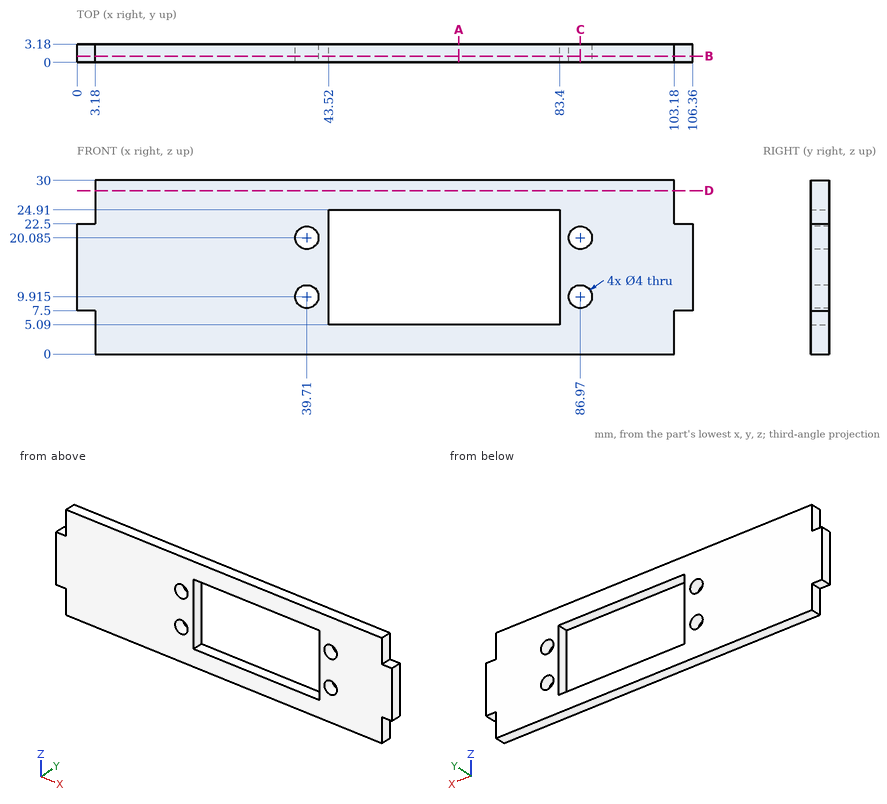
Part print with two shaded views. Sizes in mm from the minimum x, y, z corner. Round coordinates to 2 decimals unless told otherwise and drop trailing zeros. Order: outer loops, then holes, each group sorted by start corner. A loop starts at its lowest first (then second) coordinate and runs counter-clockwise, first axis right, second up.
(1) Band-saw the part on A-A (x = 66). List the corners of the cut face in (y, z).
(2) Band-saw the part on C-C (x = 86.97). List the corners of the cut face in (y, z) (3 decimals), then the cut area to 3 significant figures.
(3) Band-saw the part on D-D (z = 28.25). List the corners of the cut face in (x, y), then the cut area to 3 significant figures.
(4) Drill centre lines: line 1 (Z direction, x = 86.97, y = 1.05) (3 decimals); line 2 (Z direction, x = 81, y = 2.65); line 3 (X direction, y = 1.3, z = 15). Where is each one in solid material? Low to high.
(5) Band-saw the part on B-B (y = 1.1). List the corners of the cut face in (x, z) (3 decimals).
(6) Pin check, flat tips, straight feed: pin 1 (3 mm diameter, centred on x = 86.97, z = 9.915, fed in from +Y); pin 2 (1 mm diameter, centred on x = 2.5, y = 1.5, fed in from -Z); pin 3 (1.6 mm diameter, centred on y = 2.5, z = 5, fed in from -X). Stop position of each tip, or through.
Verdict:
1. outline: (0, 0) - (3.18, 0) - (3.18, 5.09) - (0, 5.09) - close; (0, 24.91) - (3.18, 24.91) - (3.18, 30) - (0, 30) - close
2. outline: (0, 0) - (3.18, 0) - (3.18, 7.915) - (0, 7.915) - close; (0, 11.915) - (3.18, 11.915) - (3.18, 18.085) - (0, 18.085) - close; (0, 22.085) - (3.18, 22.085) - (3.18, 30) - (0, 30) - close
2. area: 70.0 mm2
3. outline: (3.18, 0) - (103.18, 0) - (103.18, 3.18) - (3.18, 3.18) - close
3. area: 318 mm2
4. line 1: z = 0 to 7.915, 11.915 to 18.085, 22.085 to 30
4. line 2: z = 0 to 5.09, 24.91 to 30
4. line 3: x = 0 to 43.52, 83.4 to 106.36
5. outline: (0, 7.5) - (3.18, 7.5) - (3.18, 0) - (103.18, 0) - (103.18, 7.5) - (106.36, 7.5) - (106.36, 22.5) - (103.18, 22.5) - (103.18, 30) - (3.18, 30) - (3.18, 22.5) - (0, 22.5) - close; hole circle Ø4 at (39.71, 9.915); hole circle Ø4 at (39.71, 20.085); hole (43.52, 5.09) - (83.4, 5.09) - (83.4, 24.91) - (43.52, 24.91) - close; hole circle Ø4 at (86.97, 9.915); hole circle Ø4 at (86.97, 20.085)
6. pin 1: passes through
6. pin 2: stops at z = 7.5
6. pin 3: stops at x = 3.18
